Read the model definition and answer for the solid it produces. Units are mm, in the model's axes. A direction names the side the tool comes from. Give positions to 0.01 mm unless a question says otherwise; leave off trailing zeros. Write each loop counter-clockwise with the first axis right and the second up, starting at its lowest first coordinate (ties: lowest second). Pieces come first, ordered by that corner, then holes.
```python
from build123d import *

# Parameters (mm, degrees)
F0_W     = 63.5
F0_H     = 63.5
F1_DEPTH = 7.62
F3_DEPTH = 114.3
F4_SIZE2 = 19.04999
F4_SIZE  = 76.19999
F5_R     = 2.38125
F7_DEPTH = 25.4
F9_DEPTH = 25.4


# Not quite as in the source:
# - a fillet or chamfer is up to 0.001 mm smaller than in the source, because OpenCascade refuses the exact size


with BuildPart() as f1:
    # F0 (on Front) → F1 (new body)
    with BuildSketch(Plane.XZ):
        with Locations((31.75, -31.75)):
            Rectangle(F0_W, F0_H)
    extrude(amount=F1_DEPTH)

    # F2 (on face) → F3 (join)
    with BuildSketch(Plane.XZ.offset(7.62)):
        Polygon((50.8, -12.7), (31.75, -12.7), (12.7, -12.7), (12.7, -50.8), (50.8, -50.8), align=None)
    extrude(amount=F3_DEPTH)

    # F4 (size 76.2 and 19.05 in the source; OpenCascade refuses exactly that, so slightly less here)
    f4_edges = [f1.edges().sort_by_distance(p)[0] for p in [
        (31.75, -121.92, -12.7),
        (12.7, -121.92, -31.75),
        (31.75, -121.92, -50.8),
        (50.8, -121.92, -31.75),
    ]]
    chamfer(f4_edges, length=F4_SIZE, length2=F4_SIZE2)

    # F5 (on face) → F7 (cut)
    with BuildSketch(Plane.XZ.offset(7.62)):
        with Locations((6.35, -6.35)):
            Circle(F5_R)
    extrude(amount=-F7_DEPTH, mode=Mode.SUBTRACT)

    # F5 (on face) → F9 (cut)
    with BuildSketch(Plane.XZ.offset(7.62)):
        with Locations((6.35, -31.75)):
            Circle(F5_R)
        with Locations((6.35, -57.15)):
            Circle(F5_R)
        with Locations((31.75, -57.15)):
            Circle(F5_R)
        with Locations((57.15, -57.15)):
            Circle(F5_R)
        with Locations((57.15, -31.75)):
            Circle(F5_R)
        with Locations((57.15, -6.35)):
            Circle(F5_R)
        with Locations((31.75, -6.35)):
            Circle(F5_R)
    extrude(amount=-F9_DEPTH, mode=Mode.SUBTRACT)


solid = f1.part
```
Item 1: Which of the six approach directions +Z, -Z, +X, -X, +Y, -Y give full straight-line access (tool end or side, diameter ignored) to faces 1 (the flat face through (31, -26, -50.8)), 2 (the flat face through (50.8, -26, -32)), 3 (the flat face through (12.7, -26, -31))?
Result set:
face 1: -Z, +X, -X, -Y
face 2: +Z, -Z, +X, -Y
face 3: +Z, -Z, -X, -Y
Item 2: Find the intervals of material crossed by line 1 along X through (y, z) = (-3, -6); line 2 along Z through (x, y) = (57.15, -5.25); line 3 along Z through (x, y) = (31.75, -3), in increasing order.
Result set:
line 1: x = 0 to 3.99, 8.71 to 29.39, 34.11 to 54.79, 59.51 to 63.5
line 2: z = -63.5 to -59.53, -54.77 to -34.13, -29.37 to -8.73, -3.97 to 0
line 3: z = -63.5 to -59.53, -54.77 to -8.73, -3.97 to 0
Item 3: Section C-C (y = -71) is taken. Write down the section's boundary in (x, z).
Result set:
outline: (19.02, -44.48) - (44.48, -44.48) - (44.48, -19.02) - (19.02, -19.02) - close
Item 4: Determine the mould class of faces 4 (the flat face through (31.483, -75.887, -43.258)), 5 (the cylindrical face through (59.35, -3.86, -58.06)), 6 (the flat face through (43.258, -75.887, -32.017)) for opening direction X: pulls with the +X half, pulls with the -X half, needs draft (parallel to the pull), parting line crosses it, or undercut.
Result set:
face 4: needs draft
face 5: undercut
face 6: pulls with the +X half
Item 5: Section B-B (z = -57.15) is taken. Write down the section's boundary in (x, y), and give its area (3 significant figures).
Result set:
outline: (0, -7.62) - (3.97, -7.62) - (3.97, 0) - (0, 0) - close; (8.73, -7.62) - (29.37, -7.62) - (29.37, 0) - (8.73, 0) - close; (34.13, -7.62) - (54.77, -7.62) - (54.77, 0) - (34.13, 0) - close; (59.53, -7.62) - (63.5, -7.62) - (63.5, 0) - (59.53, 0) - close
area: 375 mm2
Item 6: Section A-A (x = 6.35) is taken. Write down the section's boundary in (y, z), and give its area (3 significant figures).
Result set:
outline: (-7.62, -63.5) - (0, -63.5) - (0, -59.53) - (-7.62, -59.53) - close; (-7.62, -54.77) - (0, -54.77) - (0, -34.13) - (-7.62, -34.13) - close; (-7.62, -29.37) - (0, -29.37) - (0, -8.73) - (-7.62, -8.73) - close; (-7.62, -3.97) - (0, -3.97) - (0, 0) - (-7.62, 0) - close
area: 375 mm2
Item 7: Section D-D (z = -27.5) is taken. Write down the section's boundary in (x, y), and give its area (3 significant figures).
Result set:
outline: (0, -7.62) - (12.7, -7.62) - (12.7, -45.72) - (27.5, -104.92) - (36, -104.92) - (50.8, -45.72) - (50.8, -7.62) - (63.5, -7.62) - (63.5, 0) - (0, 0) - close
area: 3,310 mm2
Item 8: Each of these flat-tipped pins is pushed along its axis until it touches: pin 1 Ø1 at (y, z) = (-36, -36.5) entering from +X; pin 2 Ø11.5 at (x, y) = (34, -20) entering from -Z; pin 3 Ø11.5 at (x, y) = (40.5, -20.5) entering from +Z. Where does it stop, or does it pass through?
Result set:
pin 1: stops at x = 50.8
pin 2: stops at z = -50.8
pin 3: stops at z = -12.7
